Autodesk Inventor part; units mm, degrees
ref_plane "YZ Plane" through (0, 0, 0) normal (1, 0, 0) x (0, 1, 0)
ref_plane "XZ Plane" through (0, 0, 0) normal (0, 1, 0) x (-1, 0, 0)
ref_plane "XY Plane" through (0, 0, 0) normal (0, 0, 1) x (1, 0, 0)
sketch "Sketch1" plane through (0, 0, 0) normal (0, 0, 1) x (1, 0, 0)
  circle A0 centre (38.1, -25.4) radius 2.1844
  circle A1 centre (84.267, 23.8448) radius 2.1844
  circle A2 centre (38.1, -25.4) radius 4.7625
  circle A3 centre (84.267, 23.8448) radius 4.7625
  line L0 (80.7926, 27.1021) -> (31.2119, -25.784)
  line L1 (36.9187, -33.6234) -> (89.3053, 22.2556)
  point P0 (0, 0)
  point P1 (34.6256, -22.1427)
  point P2 (41.5744, -28.6573)
  point P3 (87.7414, 20.5875)
  dimension "d1" = 9.525
  dimension "d0" = 9.525
extrude "Extrusion1" add sketch "Sketch1" along normal blind 6.35
properties part number "thingy"
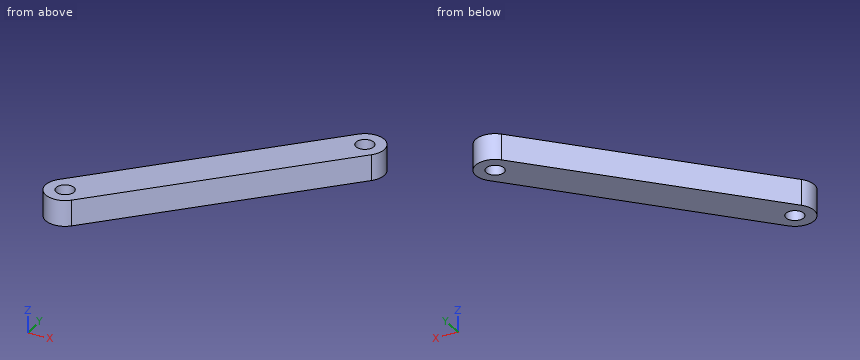
Can you work these out from the model? Positions are in its coordinate system, mm. Coordinates: 2 decimals unless noted, no trailing zeros. Order: outer loops, then holes, each group sorted by start corner. A loop starts at its lowest first (then second) coordinate and runs counter-clockwise, first axis right, second up. Notation, with made-up numbers: (15, -16.75) -> (47, -16.75) arc R22 ccw to (47, 5.25) -> close; hole circle Ø4 at (49, 41). An arc over 180 degrees is marked (long way). Write each question's results on one line, items separated by ' | '.
Item 1: If I drill on line 1 along Y through (x, z) = (38.1, 4.5); line 2 along X through (y, z) = (24.5, 5); line 3 along Y through (x, z) = (85, 6), over which ranges is the centre line in solid material (lowest first)?
Results are:
line 1: -30.16 to -27.58, -23.22 to -18.44 | line 2: 78.35 to 82.18, 86.35 to 88.98 | line 3: 17.66 to 21.79, 25.9 to 28.55
Item 2: I want a section at C-C, the plane z = 2.5. Write out the boundary of the cut face in (x, y) (1 decimal).
Results are:
outline: (34.6, -22.1) arc R4.8 ccw to (41.6, -28.7) -> (87.7, 20.6) arc R4.8 ccw to (80.8, 27.1) -> close; hole circle Ø4.4 at (38.1, -25.4); hole circle Ø4.4 at (84.3, 23.8)
Item 3: I want a section at D-D, the plane y = 12. Write out the boundary of the cut face in (x, z), then the cut area to 3 significant figures.
Results are:
outline: (66.63, 0) -> (79.69, 0) -> (79.69, 6.35) -> (66.63, 6.35) -> close | area: 82.9 mm²
Item 4: I want a section at B-B, the plane x = 38. Write out the boundary of the cut face in (y, z).
Results are:
outline: (-30.16, 0) -> (-27.58, 0) -> (-27.58, 6.35) -> (-30.16, 6.35) -> close; (-23.22, 0) -> (-18.54, 0) -> (-18.54, 6.35) -> (-23.22, 6.35) -> close
Item 5: I want a section at A-A, the plane y = 22.5. Write out the boundary of the cut face in (x, z), then the cut area to 3 significant figures.
Results are:
outline: (76.48, 0) -> (82.55, 0) -> (82.55, 6.35) -> (76.48, 6.35) -> close; (85.99, 0) -> (88.84, 0) -> (88.84, 6.35) -> (85.99, 6.35) -> close | area: 56.6 mm²
Item 6: I'm going to push flat-ended pins straight in: pin 1 Ø1 at (y, z) = (22.5, 2.5) entering from +X; pin 2 Ø3.5 at (x, y) = (38.1, -25.4) entering from +Z; pin 3 Ø1.5 at (x, z) = (75, 4) entering from +Y; pin 4 Ø5.5 at (x, y) = (84.27, 23.84) entering from -Z. Where does each tip first touch, or does it pass through?
Results are:
pin 1: x = 88.95 | pin 2: through | pin 3: y = 21.72 | pin 4: z = 0
